Answer from the drawing. Dimensions are ordinates in mm from the lowest x, y and z of the part. A direction names the side the tool comes from. Coordinates: 2 decimals unless noted, no trailing zeros. Order: outer loops, then holes, each group sorted by start corner. A loop starts at its lowest first (then second) coordinate and runs counter-clockwise, first axis right, second up.
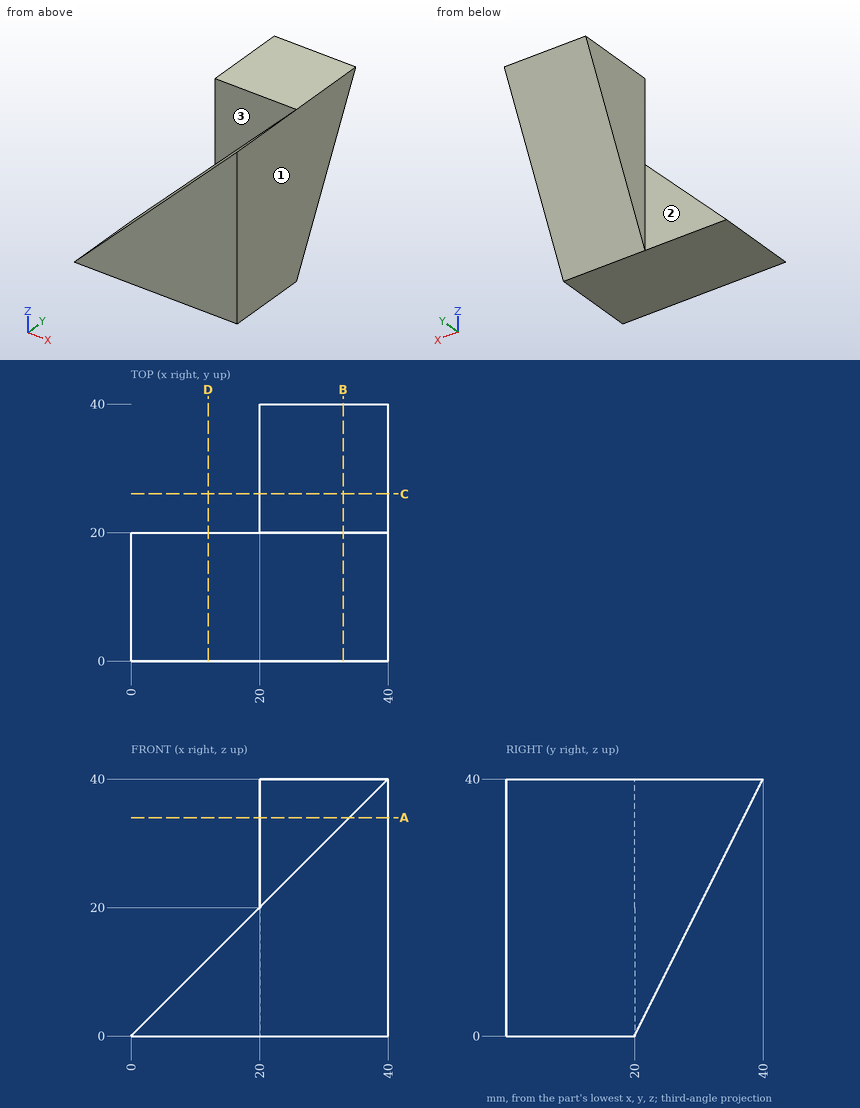
1. The part is cut by section C-C (y = 26). Determine the outline of the cut face in (x, z).
2. For the marked faces 1, 2 and 3, determine the directions among +Z, -Z, +X, -X, +Y, -Y from which every point of the face is accessible in a straight line to the end or side of a thin tool.
3. Consider probe 1 along X at (y, z) = (25.5, 32); probe 2 along X at (y, z) = (16.5, 28.5); probe 3 along Y at (x, z) = (14, 3). Determine where each line is inside the solid, lowest interval first.
4. The part is cut by section D-D (x = 12). Determine the outline of the cut face in (y, z), plus the area to 3 significant figures.
5. The part is cut by section B-B (x = 33). Determine the outline of the cut face in (y, z).
6. The part is cut by section A-A (z = 34). Determine the outline of the cut face in (x, y).
7. Flat-ended cylindrical pins translate along their axes: pin 1 (2 mm diameter, centred on x = 21.5, y = 16, fed in from +Z); pin 2 (1.5 mm diameter, centred on x = 22, z = 35.5, fed in from -Y); pin 3 (8 mm diameter, centred on x = 6.5, y = 5, fed in from +Z). Find the tip coordinate at first contact, or state that the pin passes through.
Worked out:
1. outline: (20, 12) - (40, 12) - (40, 40) - (20, 40) - close
2. face 1: +Z, -Z, +X, +Y, -Y
2. face 2: +Z, -Z, -X, +Y
2. face 3: +Z, -X, -Y
3. probe 1: x = 20 to 40
3. probe 2: x = 28.5 to 40
3. probe 3: y = 0 to 20
4. outline: (0, 0) - (20, 0) - (20, 12) - (0, 12) - close
4. area: 240 mm2
5. outline: (0, 0) - (20, 0) - (40, 40) - (20, 40) - (20, 33) - (0, 33) - close
6. outline: (20, 20) - (34, 20) - (34, 0) - (40, 0) - (40, 37) - (20, 37) - close
7. pin 1: stops at z = 22.5
7. pin 2: stops at y = 20
7. pin 3: stops at z = 10.5
